Source: CAD feature listing. Evaluate the final solid. Frame: model axes, mm. Face numbers are marked on the shaded views. A direction names the side the tool comes from. Round coordinates to 2 decimals unless told otherwise and drop trailing zeros. Write each loop counter-clockwise with the first axis right and the second up, starting at its lowest first coordinate (ties: lowest second). Pieces come first, ordered by that corner, then holes. Notation, with made-up numbers: (14.5, 13) -> (27.5, 13) arc R24 ccw to (27.5, 49) -> close; hole circle Ø4 at (66.5, 75). An arc over 180 degrees is marked (long way). Put each result on its own line as item: value.
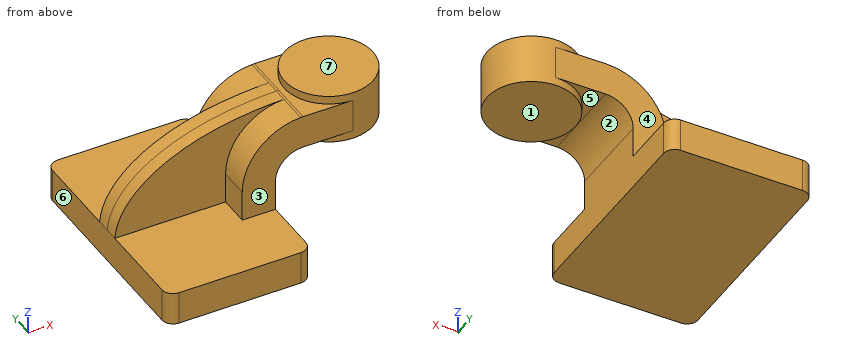
```python
from build123d import *

# Parameters (mm, degrees)
F1_DEPTH = 63.5
F2_DEPTH = 7.9375
F0_W     = 25.4
F0_H     = 19.05
F3_DEPTH = 25.4
F5_R     = 6.35


with BuildPart() as f1:
    # F0 (on Front) → F1 (new body, symmetric)
    with BuildSketch(Plane.XZ):
        Polygon((-41.275, 9.525), (-41.275, -9.525), (41.275, -9.525), (41.275, 9.525), (22.225, 9.525), align=None)
    extrude(amount=F1_DEPTH, both=True)

    # F0 (on Front) → F2 (join, symmetric)
    with BuildSketch(Plane.XZ):
        with BuildLine():
            add(Edge.make_bspline(
                [(-41.275, 9.525), (-39.6070504459, 34.3761578761), (-7.6353036908, 60.4303854768), (55.7402997063, 61.8967380816)],
                knots=[0, 0, 0, 0, 110.6868392029, 110.6868392029, 110.6868392029, 110.6868392029], degree=3))
            Line((-41.275, 9.525), (22.225, 9.525))
            Line((22.225, 9.525), (22.225, 27.0002))
            ThreePointArc((22.225, 27.0002), (31.9608216911, 51.1923665239), (55.7402997063, 61.8967380816))
        make_face()
    extrude(amount=F2_DEPTH, both=True)

    # F0 (on Front) → F3 (join, symmetric)
    with BuildSketch(Plane.XZ):
        with BuildLine():
            Line((22.225, 9.525), (41.275, 9.525))
            Line((41.275, 9.525), (41.275, 27.0002))
            ThreePointArc((41.275, 27.0002), (45.9246798487, 38.2255201513), (57.15, 42.8752))
            Line((57.15, 42.8752), (60.325, 42.8752))
            Line((60.325, 42.8752), (60.325, 61.9252))
            Line((60.325, 61.9252), (57.15, 61.9252))
            add(Edge.make_bspline(
                [(55.7402997063, 61.8967380816), (56.2084857946, 61.9075707341), (56.6783857447, 61.9170615063), (57.15, 61.9252)],
                knots=[110.6868392029, 110.6868392029, 110.6868392029, 110.6868392029, 111.5045361635, 111.5045361635, 111.5045361635, 111.5045361635], degree=3))
            ThreePointArc((55.7402997063, 61.8967380816), (31.9608216911, 51.1923665239), (22.225, 27.0002))
            Line((22.225, 27.0002), (22.225, 9.525))
        make_face()
        with Locations((73.025, 52.4002)):
            Rectangle(F0_W, F0_H)
    extrude(amount=F3_DEPTH, both=True)

    # F0 (on Front) → F4 (revolve)
    with BuildSketch(Plane.XZ):
        Polygon((85.725, 66.675), (85.725, 61.9252), (85.725, 42.8752), (85.725, 38.1), (111.125, 38.1), (111.125, 66.675), align=None)
    revolve(axis=Axis((85.725, 0, 52.3875), (0, 0, -1)))

    # F5
    f5_edges = [f1.edges().sort_by_distance(p)[0] for p in [
        (41.275, -63.5, 0),
        (-41.275, -63.5, 0),
        (41.275, 63.5, 0),
        (-41.275, 63.5, 0),
    ]]
    fillet(f5_edges, radius=F5_R)


solid = f1.part
```
Q1. Reachability of the marked faces 1, 2, 3 and 4 from +Z, -Z, +X, -X, +Y, -Y: full face, straight path, thin tool, end or side. Return the list, or none.
Ans:
face 1: -Z, +X, +Y, -Y
face 2: -Z, +Y, -Y
face 3: +Z, +X, -X, -Y
face 4: +Z, +X, -X, +Y
Q2. Pin query (flat end, axial travel): pin 1 (1 mm diameter, centred on x = 43, z = 41, fed in from -Y); pin 2 (23 mm diameter, centred on x = 76.5, y = 3, fed in from -Z); pin 3 (1.5 mm diameter, centred on y = 24, z = 22.5, fed in from -X) (3 decimals). Return the tip coordinate at first contact, or that it passes through.
Ans:
pin 1: stops at y = -25.4
pin 2: stops at z = 38.1
pin 3: stops at x = 22.225
Q3. Cut plane B-B on x = 78.5. Output: boundary loops of the cut face in (y, z) (3 decimals), and give its area (3 significant figures).
Ans:
outline: (-25.4, 42.875) -> (-24.351, 42.875) -> (-24.351, 38.1) -> (24.351, 38.1) -> (24.351, 42.875) -> (25.4, 42.875) -> (25.4, 61.925) -> (24.351, 61.925) -> (24.351, 66.675) -> (-24.351, 66.675) -> (-24.351, 61.925) -> (-25.4, 61.925) -> close
area: 1,430 mm^2
Q4. Cut plane A-A on z = 6. Output: boundary loops of the cut face in (x, y) (3 decimals).
Ans:
outline: (-41.275, -57.15) arc R6.35 ccw to (-34.925, -63.5) -> (34.925, -63.5) arc R6.35 ccw to (41.275, -57.15) -> (41.275, 57.15) arc R6.35 ccw to (34.925, 63.5) -> (-34.925, 63.5) arc R6.35 ccw to (-41.275, 57.15) -> close
Q5. Draft query along X for the marked faces 5, 6 and 7. Return one class per face: +X half, -X half, draft (parallel to the pull), parting line (faces both ways), or undercut.
Ans:
face 5: undercut
face 6: -X half
face 7: draft
Q6. Cut plane C-C on y = -29. Output: boundary loops of the cut face in (x, z) (3 decimals).
Ans:
outline: (-41.275, -9.525) -> (41.275, -9.525) -> (41.275, 9.525) -> (-41.275, 9.525) -> close
Q7. Material intervals for line 1 (Y direction, x = 28, z = 17); line 2 (Z direction, x = 17, y = 34) (3 decimals); line 3 (Z direction, x = 83, y = 1.5) (3 decimals), sorted ascending. Write a range as [from, to].
Ans:
line 1: y = [-25.4, 25.4]
line 2: z = [-9.525, 9.525]
line 3: z = [38.1, 66.675]
